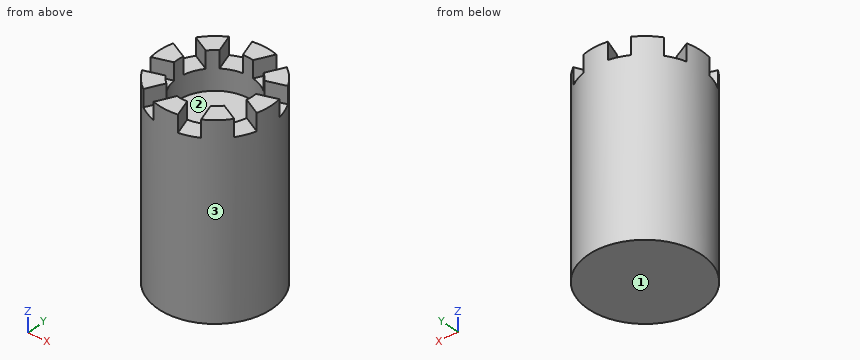
```python
from build123d import *

# Parameters (mm, degrees)
BOX_W               = 20
BOX_H               = 10
BOX_DEPTH           = 10
BOX_PLACEMENT_ANGLE = 18
ARRAY_COUNT         = 8
CYLINDER001_R       = 20
CYLINDER001_DEPTH   = 20
CYLINDER_R          = 30
CYLINDER_DEPTH      = 100


with BuildPart() as rectangles:
    # Box → Box (new body)
    with BuildSketch(Plane.XY):
        with Locations((10, 5)):
            Rectangle(BOX_W, BOX_H)
    extrude(amount=BOX_DEPTH)


with BuildPart() as rectangles_1:
    # Box placement: moved
    add(rectangles.part.moved(Location((14, 0, 91))).rotate(Axis((14, 0, 91), (0, 0, 1)), BOX_PLACEMENT_ANGLE))

    # Array: Rectangles ×8 about axis
    array_axis = Axis((0, 0, 0), (0, 0, 1))


with BuildPart() as rectangles_2:
    add(rectangles_1.part)
    for i in range(1, ARRAY_COUNT):
        add(rectangles_1.part.rotate(array_axis, i * 360 / ARRAY_COUNT))


with BuildPart() as cilindre001:
    # Cylinder001 → Cylinder001 (new body)
    with BuildSketch(Plane.XY.offset(80)):
        Circle(CYLINDER001_R)
    extrude(amount=CYLINDER001_DEPTH)


with BuildPart() as obj1:
    # Cylinder → Cylinder (new body)
    with BuildSketch(Plane.XY):
        Circle(CYLINDER_R)
    extrude(amount=CYLINDER_DEPTH)

    # Cut: cut Cilindre001
    add(cilindre001.part, mode=Mode.SUBTRACT)

    # Cut001: cut Rectangles
    add(rectangles_2.part, mode=Mode.SUBTRACT)


solid = obj1.part
```
CAD build for the part. Positions are in the model's coordinates, mm. Face numbers are marked on the shaded views. Give positions to 0.01 mm unless a question says otherwise; leave off trailing zeros. Order: outer loops, then holes, each group sorted by start corner. A loop starts at its lowest first (then second) coordinate and runs counter-clockwise, first axis right, second up. Notation, with made-up numbers: M 79,52 L 135,52 A30 ccw 135,86 Z; hole C 10,-4.5 d4. An arc over 180 degrees is marked long. Put each result on its own line as item: value. Start each with the question number.
(1) Flat gauge pins, fed straight in: pin 1 Ø4 at (x, y) = (-9, 21.5) entering from +Z; pin 2 Ø10 at (y, z) = (-13.5, 16.5) entering from +X; pin 3 Ø14 at (x, y) = (-21.5, -7) entering from +Z; pin 4 Ø10 at (x, z) = (-1.5, 28.5) entering from -Y. Where does each tip first touch, or does it go through?
(2) Saw through at A-A, the plane y = 0. Write the cut outline in (x, z).
(3) Mould opens along Y. For the marked faces 1, 2 and 3 say: +Y half, -Y half, draft (parallel to the pull), parting line (faces both ways), or undercut.
(4) Saw through at C-C, the plane z = 72. Write the cut outline in (x, y), then the cut area to 3 significant figures.
(5) Drill centre lines: line 1 along X through (y, z) = (0, 86); line 2 along Y through (x, z) = (0, 55). Where is each one in solid material? Low to high.
Check result:
1. pin 1: stops at z = 91
1. pin 2: stops at x = 28.77
1. pin 3: stops at z = 100
1. pin 4: stops at y = -30
2. outline: M -30,0 L 30,0 L 30,100 L 20,100 L 20,80 L -20,80 L -20,100 L -30,100 Z
3. face 1: draft
3. face 2: undercut
3. face 3: parting line
4. outline: C 0,0 d60
4. area: 2,830 mm2
5. line 1: x = -30 to -20, 20 to 30
5. line 2: y = -30 to 30
